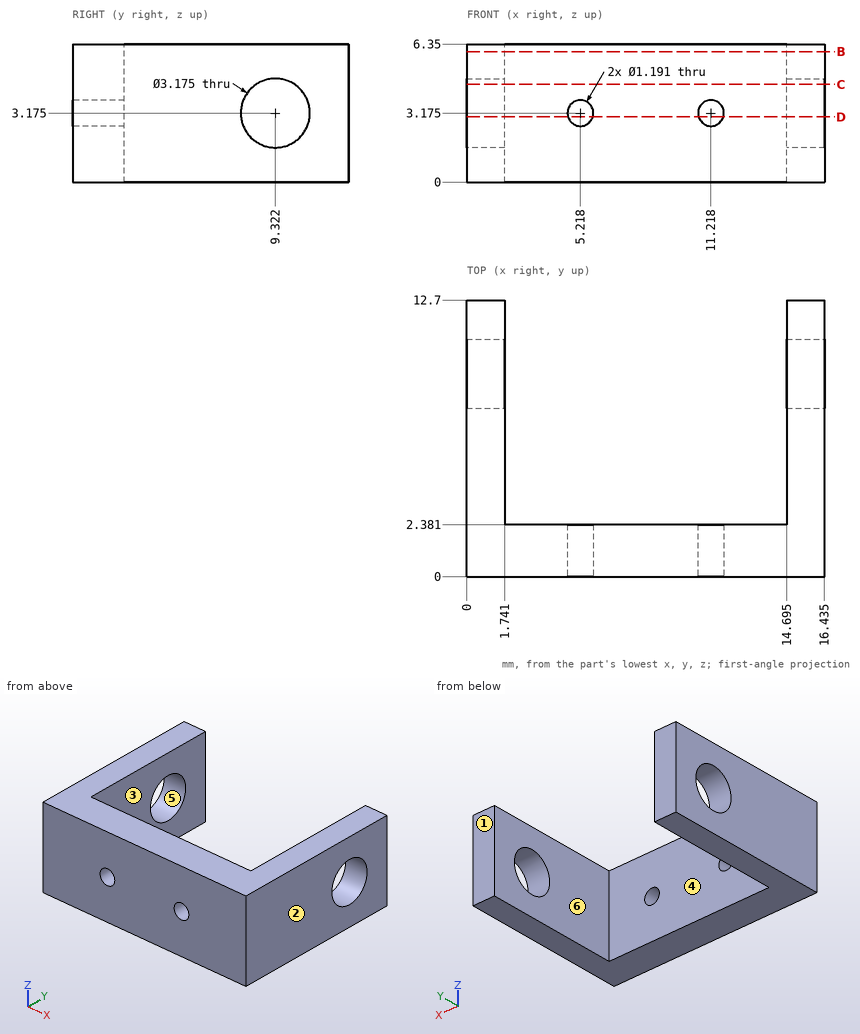
Drawing for the job (mm, zero at the part's lowest x, y, z). A direction names the side the tool comes from. Round coordinates to 2 decimals unless told otherwise and drop trailing zeros. Loops run counter-clockwise (first coordinate to the right, second up) from the corner with the lowest first, then second, coordinate; pieces in that order, holes last. Notation, with made-up numbers: (89, -17.5) -> (144, -17.5) arc R21 ccw to (144, 21.5) -> close; hole circle Ø6 at (15, 18.5). An arc over 180 degrees is marked (long way). Answer as CSV lines item,"result". Start each with the question number.
1) Probe line 1 along X through (y, z) = (4, 0.75) (1 decimal); line 2 along Z through (x, y) = (5.25, 0.5); line 3 along Y through (x, z) = (7.75, 1.5). List the from-to ranges inside material, lowest first.
2) Tool access for the marked faces 5 and 6: list every direction of +Z, -Z, +X, -X, +Y, -Y with a clear straight run to the whole face (end or side of a thin tool).
3) Pin check, flat tips, straight feed: P1, Ø1.4, axis at x = 11.22, z = 3.18, coming from the -Y side; P2, Ø1.9, axis at x = 5.22, z = 3.18, coming from the +Y side. Stop position of each tip, or through.
4) Slice it at D-D (z = 3). List the corners of the cut face in (x, y) (1 decimal).
5) Slice it at B-B (z = 6). List the corners of the cut face in (x, y) (1 decimal).
6) Slice it at C-C (z = 4.5). List the corners of the cut face in (x, y) (1 decimal).
7) Mould opens along X. For the marked faces 1, 2, 3 and 4 say: +X half, -X half, draft (parallel to the pull), parting line (faces both ways), or undercut.
Filled in:
1,line 1,"x = 0 to 1.7, 14.7 to 16.4"
1,line 2,"z = 0 to 2.58, 3.77 to 6.35"
1,line 3,"y = 0 to 2.38"
2,face 5,"+X, -X"
2,face 6,"+Z, -Z, +Y"
3,P1,"stops at y = 0"
3,P2,"stops at y = 2.38"
4,outline,"(0, 0) -> (4.6, 0) -> (4.6, 2.4) -> (1.7, 2.4) -> (1.7, 7.7) -> (0, 7.7) -> close; (0, 10.9) -> (1.7, 10.9) -> (1.7, 12.7) -> (0, 12.7) -> close; (5.8, 0) -> (10.6, 0) -> (10.6, 2.4) -> (5.8, 2.4) -> close; (11.8, 0) -> (16.4, 0) -> (16.4, 7.7) -> (14.7, 7.7) -> (14.7, 2.4) -> (11.8, 2.4) -> close; (14.7, 10.9) -> (16.4, 10.9) -> (16.4, 12.7) -> (14.7, 12.7) -> close"
5,outline,"(0, 0) -> (16.4, 0) -> (16.4, 12.7) -> (14.7, 12.7) -> (14.7, 2.4) -> (1.7, 2.4) -> (1.7, 12.7) -> (0, 12.7) -> close"
6,outline,"(0, 0) -> (16.4, 0) -> (16.4, 8.4) -> (14.7, 8.4) -> (14.7, 2.4) -> (1.7, 2.4) -> (1.7, 8.4) -> (0, 8.4) -> close; (0, 10.2) -> (1.7, 10.2) -> (1.7, 12.7) -> (0, 12.7) -> close; (14.7, 10.2) -> (16.4, 10.2) -> (16.4, 12.7) -> (14.7, 12.7) -> close"
7,face 1,"draft"
7,face 2,"+X half"
7,face 3,"undercut"
7,face 4,"undercut"
